Job drawing, mm, ordinate dimensions from the low corner. One solid piece. Coordinates: 2 decimals unless noted, no trailing zeros. Order: outer loops, then holes, each group sorted by start corner. A loop starts at its lowest first (then second) coordinate and runs counter-clockwise, first axis right, second up. Notation, with made-up numbers: (48, 13.5) - (67, 13.5) arc R25 cw to (67, 32.5) - close; hole circle Ø8 at (-1.5, 74). An arc over 180 degrees is marked (long way). Return JSON: item names as keys, results as strings.
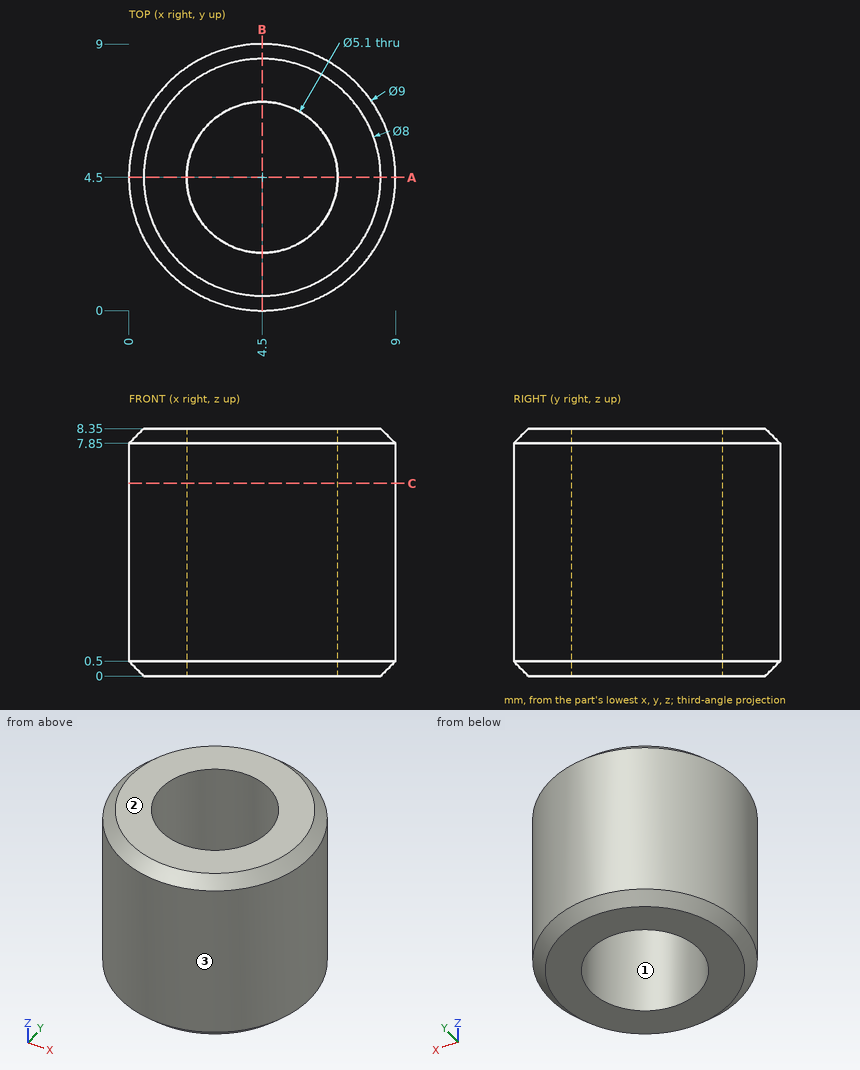
1. Cut at C-C on z = 6.5. Give the cut face in (x, y), plus the area to 3 significant figures.
Check values:
{"outline": "circle Ø9 at (4.5, 4.5); hole circle Ø5.1 at (4.5, 4.5)", "area": "43.2 mm²"}
2. Probe L1, parallel to Y at x = 4.5, z = 6.25; L2, parallel to Y at x = 6, z = 8.25; L3, parallel to X at y = 2.5, z = 2.25. List the from-to ranges inside material, lowest first.
Check values:
{"L1": "0 to 1.95, 7.05 to 9", "L2": "0.68 to 2.44, 6.56 to 8.32", "L3": "0.47 to 2.92, 6.08 to 8.53"}
3. Mould opens along X. For the marked faces 1, 2 and 3 say: pulls with the +X half, pulls with the -X half, needs draft (parallel to the pull), parting line crosses it, or undercut.
Check values:
{"face 1": "undercut", "face 2": "needs draft", "face 3": "parting line crosses it"}
4. Cut at A-A on y = 4.5. Give the cut face in (x, z), plus the area to 3 significant figures.
Check values:
{"outline": "(0, 0.5) - (0.5, 0) - (1.95, 0) - (1.95, 8.35) - (0.5, 8.35) - (0, 7.85) - close; (7.05, 0) - (8.5, 0) - (9, 0.5) - (9, 7.85) - (8.5, 8.35) - (7.05, 8.35) - close", "area": "32.1 mm²"}
5. Drop flat-ended pins along their axis: pin 1 (2 mm diameter, centred on x = 1.5, z = 3.5, fed in from +Y); pin 2 (1.5 mm diameter, centred on x = 5.5, z = 7, fed in from -Y); pin 3 (2 mm diameter, centred on y = 1, z = 2.5, fed in from -X). Give the stop position or say it passes through.
Check values:
{"pin 1": "y = 8.53", "pin 2": "y = 0.01", "pin 3": "x = 0.76"}
